Input: part model. Units: mm. Frame: model coordinates. A direction names the side the tool comes from. Give positions to 0.01 mm unless a question says otherwise; leave off trailing zeros. Loops run counter-clockwise (first coordinate to the right, second up) from the corner with the lowest first, then second, coordinate; pieces in that order, holes last. Notation, with made-up numbers: M 49,65 L 57,65 A22 ccw 57,87 Z; hole C 67,-13 d6. An arc over 180 degrees is marked long. Answer as a JSON object with one key per item and string values. Group by question number.
1) Ray query, L1, parallel to Y at x = -14.5, z = 9.5; L2, parallel to Y at x = 16, z = 8.5; L3, parallel to X at y = -3.5, z = 6.5. Return the intervals inside material, ascending.
2) Draft query along Y for faces 1 (the flat face through (6, 0, 10)), 2 (the flat face through (1.643, 29.763, 4.93)), 3 (the cylindrical face through (6.75, -9.32, 4.93)). Return one class per face: +Y half, -Y half, draft (parallel to the pull), parting line (faces both ways), or undercut.
3) Section query D-D on x = -21.5. Return loops of the section in (y, z).
4) Section query B-B on y = 18.5. Return loops of the section in (x, z), plus the area to 3 significant figures.
5) Access query for faces 4 (the flat face through (-1.64, 29.74, 4.93)), 5 (the cylindrical face through (-1.393, -13.815, 4.93)). Directions: +Z, -Z, +X, -X, +Y, -Y. A direction counts if a zero-diameter tool reaches every point of the face in a straight line with its end or side. Return the directions, or none.
6) First-contact query: P1, Ø5, axis at x = -20.5, z = 7, coming from the -Y side; P2, Ø2, axis at x = 16.5, z = 4.5, coming from the +Y side; P3, Ø4, axis at x = -21, z = 3, coming from the -Y side. Flat tips, straight axial feed; report the tip coordinate or a pass-through.
7) Section query A-A on x = 0. Return loops of the section in (y, z).
8) Section query C-C on y = -12. Return loops of the section in (x, z).
from build123d import *

# Parameters (mm, degrees)
SZKIC1_R                    = 4.5
SZKIC1_R_2                  = 6.5
DODANIE_WYCI_GNI_CIE1_DEPTH = 10


with BuildPart() as part:
    # Szkic1 → Dodanie-wyciągnięcie1 (new body)
    with BuildSketch(Plane.XY):
        with BuildLine():
            Line((1.680612664, 30.453662195), (1.603352408, 29.053662195))
            ThreePointArc((1.603352408, 29.053662195), (0, 27.536352592), (-1.603352408, 29.053662195))
            Line((-1.603352408, 29.053662195), (-1.680612664, 30.453662195))
            ThreePointArc((-1.680612664, 30.453662195), (0, -30.5), (1.680612664, 30.453662195))
        make_face()
        Circle(SZKIC1_R, mode=Mode.SUBTRACT)
        with Locations((0, 17.5)):
            Circle(SZKIC1_R_2, mode=Mode.SUBTRACT)
        with Locations((13.682050943, 10.911071533)):
            Circle(SZKIC1_R_2, mode=Mode.SUBTRACT)
        with Locations((17.061238463, -3.894116344)):
            Circle(SZKIC1_R_2, mode=Mode.SUBTRACT)
        with Locations((7.592965435, -15.766955188)):
            Circle(SZKIC1_R_2, mode=Mode.SUBTRACT)
        with Locations((-7.592965435, -15.766955188)):
            Circle(SZKIC1_R_2, mode=Mode.SUBTRACT)
        with Locations((-17.061238463, -3.894116344)):
            Circle(SZKIC1_R_2, mode=Mode.SUBTRACT)
        with Locations((-13.682050943, 10.911071533)):
            Circle(SZKIC1_R_2, mode=Mode.SUBTRACT)
    extrude(amount=DODANIE_WYCI_GNI_CIE1_DEPTH)


solid = part.part
Output:
{
 "1": {"L1": "y = -26.83 to -9.87, 2.08 to 4.46, 17.36 to 26.83", "L2": "y = -25.97 to -10.31, 2.52 to 4.84, 16.98 to 25.97", "L3": "x = -30.3 to -23.55, -10.57 to -2.83, 2.83 to 10.57, 23.55 to 30.3"},
 "2": {"face 1": "draft", "face 2": "+Y half", "face 3": "undercut"},
 "3": {"outline": "M -21.63,0 L -8.64,0 L -8.64,10 L -21.63,10 Z; M 0.85,0 L 21.63,0 L 21.63,10 L 0.85,10 Z"},
 "4": {"outline": "M -24.25,0 L -6.42,0 L -6.42,10 L -24.25,10 Z; M 6.42,0 L 24.25,0 L 24.25,10 L 6.42,10 Z", "area": "357 mm^2"},
 "5": {"face 4": "+Z, -Z, +Y", "face 5": "+Z, -Z"},
 "6": {"P1": "stops at y = -24.62", "P2": "stops at y = 26.27", "P3": "stops at y = -23.86"},
 "7": {"outline": "M -30.5,0 L -4.5,0 L -4.5,10 L -30.5,10 Z; M 4.5,0 L 11,0 L 11,10 L 4.5,10 Z; M 24,0 L 27.54,0 L 27.54,10 L 24,10 Z"},
 "8": {"outline": "M -28.04,0 L -12.89,0 L -12.89,10 L -28.04,10 Z; M -2.3,0 L 2.3,0 L 2.3,10 L -2.3,10 Z; M 12.89,0 L 28.04,0 L 28.04,10 L 12.89,10 Z"}
}
